Here's how the part is built. I have some questions about the finished solid (model axes, mm). A direction names the side the tool comes from. Give positions to 0.01 mm unless a question says otherwise; leave off trailing zeros. Loops run counter-clockwise (first coordinate to the right, second up) from the corner with the lowest first, then second, coordinate; pieces in that order, holes last. Notation, with made-up numbers: (10, 73.25) - (55, 73.25) arc R8 cw to (55, 78.25) - close; hole circle Ø2 at (3, 83). An arc over 180 degrees is marked (long way). Return JSON: item names as keys, results as strings. Group by question number.
(1) I need wall thicknesses on probe 1 along Z at (x, y) = (1.75, 0); probe 2 along Z at (x, y) = (2.25, 0). Which ranges of each line are inside material? Lowest first, please. Write a range as [from, to].
(2) If we section it at A-A (z = 0): Please give me the cut outline in (x, y), then the cut area to 3 significant figures.
(3) If we section it at C-C (x = 1): Please give me the cut outline in (y, z) (1 decimal), then the cut area to 3 significant figures.
(4) On a 3-axis mill with a long thin cutter (end or side, diameter ignored), from which of +Z, -Z, +X, -X, +Y, -Y can I reach the whole of each face in a straight line? I mean faces 1 (the cylindrical face through (-0.62, 10.6, -3.34)), 2 (the flat face through (-3.556, -5, 2)). Say none if no direction works.
(5) If we mould it in two halves opening along Z, with no side actions, what happens to faces 3 (the flat face through (3.556, 5, 0)), 4 (the cylindrical face through (-0.05, -3.78, 2.9)), 5 (the cylindrical face through (2.78, 11.81, -3.72))? For each: released by +Z, released by -Z, zero draft, split by the parting line, or undercut.
(6) For P1, Ø8.5, axis at y = 0, z = 0, coming from the +X side; P2, Ø1.5, axis at x = 2, z = -8.5, coming from the +Y side; P3, Ø1.5, axis at x = -2.5, y = -9.5, coming from the +Z side, each with a flat end and sliding along its axis, tell me the tip position at first contact or that it passes through.
```python
from build123d import *

# Parameters (mm, degrees)
CHAMFER1_SIZE = 0.254


with BuildPart() as part:
    # Sketch1 → Revolve1 (revolve)
    with BuildSketch(Plane.XY):
        Polygon((-3.556, 11.1125), (1.9812, 11.1125), (1.9812, 12.3825), (3.556, 12.3825), (3.556, 4.7625), (-3.556, 4.7625), align=None)
    revolve(axis=Axis((3.556, 0, 0), (-1, 0, 0)))

    # Chamfer1
    chamfer1_edges = [part.edges().sort_by_distance(p)[0] for p in [
        (-3.556, -11.1125, 0),
        (1.9812, -12.3825, 0),
        (3.556, -12.3825, 0),
    ]]
    chamfer(chamfer1_edges, length=CHAMFER1_SIZE)


solid = part.part
```
Values:
{
 "1": {"probe 1": "[-11.11, -4.76], [4.76, 11.11]", "probe 2": "[-12.38, -4.76], [4.76, 12.38]"},
 "2": {"outline": "(-3.56, -10.86) - (-3.3, -11.11) - (1.98, -11.11) - (1.98, -12.13) - (2.24, -12.38) - (3.3, -12.38) - (3.56, -12.13) - (3.56, -4.76) - (-3.56, -4.76) - close; (-3.56, 4.76) - (3.56, 4.76) - (3.56, 12.13) - (3.3, 12.38) - (2.24, 12.38) - (1.98, 12.13) - (1.98, 11.11) - (-3.3, 11.11) - (-3.56, 10.86) - close", "area": "94.1 mm2"},
 "3": {"outline": "circle Ø22.2 at (0, 0); hole circle Ø9.5 at (0, 0)", "area": "317 mm2"},
 "4": {"face 1": "-X", "face 2": "+Z, -Z, -X, +Y, -Y"},
 "5": {"face 3": "zero draft", "face 4": "undercut", "face 5": "split by the parting line"},
 "6": {"P1": "through", "P2": "y = 9.63", "P3": "z = 6.85"}
}
